```python
from build123d import *

# Parameters (mm, degrees)
BOSS_EXTRU_1_DEPTH      = 75
CONG_1_R                = 5
ESQUISSE2_W             = 12
ESQUISSE2_H             = 27
BOSS_EXTRU_2_DEPTH      = 1.5
ESQUISSE3_R             = 14
ENL_V_MAT_EXTRU_1_DEPTH = 87.989941947
ENL_V_MAT_EXTRU_2_DEPTH = 94.429117653
ENL_V_MAT_EXTRU_3_DEPTH = 89.887569593
ESQUISSE6_R             = 1.2
ENL_V_MAT_EXTRU_4_DEPTH = 20
ESQUISSE7_R             = 1.2
ENL_V_MAT_EXTRU_5_DEPTH = 89.46044325
ESQUISSE9_W             = 15
ESQUISSE9_H             = 10
BOSS_EXTRU_3_DEPTH      = 30
CONG_2_R                = 10
CONG_3_R                = 5
ESQUISSE10_R            = 1.2
ENL_V_MAT_EXTRU_6_DEPTH = 10
ESQUISSE11_R            = 1.2
ENL_V_MAT_EXTRU_7_DEPTH = 15
ESQUISSE12_W            = 12
ESQUISSE12_H            = 2.5
ENL_V_MAT_EXTRU_8_DEPTH = 159.113883129


with BuildPart() as part:
    # Esquisse1 → Boss.-Extru.1 (new, symmetric)
    with BuildSketch(Plane.XY):
        Polygon((-12, 0), (0, 0), (0, 1.5), (5, 1.5), (23, 20), (28, 20), (28, 18.5), (40, 18.5), (40, 12.5), (24.074103459, 12.5), (6.074103459, -6), (-12, -6), align=None)
    extrude(amount=BOSS_EXTRU_1_DEPTH, both=True)

    # Congé1
    cong_1_edges = [part.edges().sort_by_distance(p)[0] for p in [
        (5, 1.5, 0),
        (23, 20, 0),
        (40, 12.5, 0),
        (24.074103459, 12.5, 0),
        (6.074103459, -6, 0),
        (-12, -6, 0),
    ]]
    fillet(cong_1_edges, radius=CONG_1_R)

    # Esquisse2 → Boss.-Extru.2 (add)
    with BuildSketch(Plane(origin=(0, 0, 0), x_dir=(1, 0, 0), z_dir=(0, 1, 0))):
        with Locations((-6, -4)):
            Rectangle(ESQUISSE2_W, ESQUISSE2_H)
    extrude(amount=BOSS_EXTRU_2_DEPTH)

    # Esquisse3 → Enlèv. mat.-Extru.1 (cut, through all)
    with BuildSketch(Plane(origin=(0, 1.5, 0), x_dir=(1, 0, 0), z_dir=(0, 1, 0))):
        with Locations((-14, -4)):
            Circle(ESQUISSE3_R)
    extrude(amount=-ENL_V_MAT_EXTRU_1_DEPTH, mode=Mode.SUBTRACT)

    # Esquisse4 → Enlèv. mat.-Extru.2 (cut, through all)
    with BuildSketch(Plane(origin=(40, 0, 0), x_dir=(0, 0, -1), z_dir=(1, 0, 0))):
        with BuildLine():
            Line((-22, 12), (-18, 9))
            ThreePointArc((-18, 9), (0, 3), (18, 9))
            Line((18, 9), (22, 12))
            ThreePointArc((22, 12), (24.208203932, 14.645898034), (25, 18))
            Line((25, 18), (25, 20))
            Line((25, 20), (-25, 20))
            Line((-25, 20), (-25, 18))
            ThreePointArc((-25, 18), (-24.208203932, 14.645898034), (-22, 12))
        make_face()
    extrude(amount=-ENL_V_MAT_EXTRU_2_DEPTH, mode=Mode.SUBTRACT)

    # Esquisse5 → Enlèv. mat.-Extru.3 (cut, through all)
    with BuildSketch(Plane(origin=(0, 20, 0), x_dir=(1, 0, 0), z_dir=(0, 1, 0))):
        with BuildLine():
            Line((40, 25), (31.163059803, 25))
            ThreePointArc((31.163059803, 25), (26.361328616, 23.849850491), (22.601776236, 20.649033065))
            Line((22.601776236, 20.649033065), (22.601776236, -20.649033065))
            ThreePointArc((22.601776236, -20.649033065), (26.361328616, -23.849850491), (31.163059803, -25))
            Line((31.163059803, -25), (40, -25))
            Line((40, -25), (40, 25))
        make_face()
    extrude(amount=-ENL_V_MAT_EXTRU_3_DEPTH, mode=Mode.SUBTRACT)

    # Esquisse6 → Enlèv. mat.-Extru.4 (cut)
    with BuildSketch(Plane.XY.offset(75)):
        with Locations((25, 16)):
            Circle(ESQUISSE6_R)
        with Locations((5, -2.5)):
            Circle(ESQUISSE6_R)
    enl_v_mat_extru_4 = extrude(amount=-ENL_V_MAT_EXTRU_4_DEPTH, mode=Mode.SUBTRACT)

    # Esquisse7 → Enlèv. mat.-Extru.5 (cut, through all)
    with BuildSketch(Plane(origin=(0, 18.5, 0), x_dir=(1, 0, 0), z_dir=(0, 1, 0))):
        with Locations(Location((35, -55, 0), (0, 0, 180))):
            Circle(ESQUISSE7_R)
        with Locations(Location((-7, -55, 0), (0, 0, 90))):
            Circle(ESQUISSE7_R)
    enl_v_mat_extru_5 = extrude(amount=-ENL_V_MAT_EXTRU_5_DEPTH, mode=Mode.SUBTRACT)

    # Symétrie1: Enlèv. mat.-Extru.4, Enlèv. mat.-Extru.5 across plane
    add(enl_v_mat_extru_4.mirror(Plane.XY), mode=Mode.SUBTRACT)
    add(enl_v_mat_extru_5.mirror(Plane.XY), mode=Mode.SUBTRACT)

    # Esquisse9 → Boss.-Extru.3 (add)
    with BuildSketch(Plane(origin=(0, 0, 0), x_dir=(1, 0, 0), z_dir=(0, 1, 0))):
        with Locations((-14.5, 34.5)):
            Rectangle(ESQUISSE9_W, ESQUISSE9_H)
    extrude(amount=-BOSS_EXTRU_3_DEPTH)

    # Congé2
    cong_2_edges = [part.edges().sort_by_distance(p)[0] for p in [
        (-7, -6, -34.5),
        (-7, -30, -34.5),
    ]]
    fillet(cong_2_edges, radius=CONG_2_R)

    # Congé3
    cong_3_edges = [part.edges().sort_by_distance(p)[0] for p in [
        (-12, -0.5, -39.5),
        (-10.535533906, -4.535533906, -39.5),
        (-2, -6, -39.5),
    ]]
    fillet(cong_3_edges, radius=CONG_3_R)

    # Esquisse10 → Enlèv. mat.-Extru.6 (cut)
    with BuildSketch(Plane.XY.offset(-29.5)):
        with Locations((-18, -24)):
            Circle(ESQUISSE10_R)
        with Locations((-18, -6)):
            Circle(ESQUISSE10_R)
    extrude(amount=-ENL_V_MAT_EXTRU_6_DEPTH, mode=Mode.SUBTRACT)

    # Esquisse11 → Enlèv. mat.-Extru.7 (cut)
    with BuildSketch(Plane(origin=(0, 0, 0), x_dir=(1, 0, 0), z_dir=(0, 1, 0))):
        with Locations(Location((-14, 34.5, 0), (0, 0, 270))):
            Circle(ESQUISSE11_R)
    extrude(amount=-ENL_V_MAT_EXTRU_7_DEPTH, mode=Mode.SUBTRACT)

    # Esquisse12 → Enlèv. mat.-Extru.8 (cut, through all)
    with BuildSketch(Plane.XY.offset(75)):
        with Locations((34, 18.75)):
            Rectangle(ESQUISSE12_W, ESQUISSE12_H)
    extrude(amount=-ENL_V_MAT_EXTRU_8_DEPTH, mode=Mode.SUBTRACT)


solid = part.part
```
Source: CAD feature listing. Evaluate the final solid. Frame: model axes, mm. A direction names the side the tool comes from. Give positions to 0.01 mm unless a question says otherwise; leave off trailing zeros. Write each loop counter-clockwise with the first axis right and the second up, starting at its lowest first coordinate (ties: lowest second). Pieces come first, ordered by that corner, then holes.
1. Section query B-B (y = -12.5). Return the cut outline in (x, z).
2. Section query C-C (z = -14.5). Return the cut outline in (x, y), then the cut area to 3 significant figures.
3. Material intervals for line 1 along Z through (x, y) = (35, 14.5); line 2 along Y through (x, z) = (3, 63); line 3 along X through (y, z) = (14.05, 55), sorted ascending.
4. Access query for faces 1 (the face through (-10, -5, 46)), 2 (the face through (36, 15, 25)), 3 (the face through (-16, -18, -39.5)), 4 (the face through (31, 12.5, 50)). Directions: +Z, -Z, +X, -X, +Y, -Y. A direction counts if a zero-diameter tool reaches every point of the face in a straight line with its end or side. Return the directions, or none.
5. First-contact query: pin 1 (0.5 mm diameter, centred on y = -0.5, z = -19.5, fed in from -X); pin 2 (0.7 mm diameter, centred on x = 5, y = -2.5, fed in from +Z); pin 3 (0.8 mm diameter, centred on y = 0.5, z = 38, fed in from -X). Flat tips, straight axial feed; report the tip coordinate or a pass-through.
6. Pull-direction query (Z, two-part tool) for faces 5 (the face through (-10.01, -27.15, -34.57)), 6 (the face through (23, 14.602, -24.186)), 7 (the face through (-13.5, -0.51, -40.93)); classes: +Z half, -Z half, draft (parallel to the pull), parting line (faces both ways), or undercut.
7. Section query A-A (z = 33). Return the cut outline in (x, y), then the cut area to 3 significant figures.
Output values:
1. outline: (-22, -39.5) - (-6.37, -39.5) - (-6.37, -29.5) - (-22, -29.5) - close; hole circle Ø2.4 at (-14, -34.5)
2. outline: (-12, -1) arc R5 ccw to (-7, -6) - (3.96, -6) arc R5 ccw to (7.55, -4.49) - (18.47, 6.74) - (10.1, 6.74) - (6.47, 3.01) arc R5 cw to (2.89, 1.5) - (0, 1.5) - (0, 0) - (-12, 0) - close
2. area: 183 mm2
3. line 1: z = -75 to -56.2, -53.8 to -25, 25 to 53.8, 56.2 to 75
3. line 2: y = -6 to 1.5
3. line 3: x = 17.21 to 33.8, 36.2 to 38.62
4. face 1: +Z, -X, -Y
4. face 2: +X, +Y, -Y
4. face 3: -Z, -X, -Y
4. face 4: +Z, -Z, +X, -Y
5. pin 1: stops at x = -12
5. pin 2: stops at z = 55
5. pin 3: stops at x = 0
6. face 5: draft
6. face 6: undercut
6. face 7: -Z half
7. outline: (-12, -1) arc R5 ccw to (-7, -6) - (3.96, -6) arc R5 ccw to (7.55, -4.49) - (22.6, 10.99) arc R5 cw to (26.19, 12.5) - (35, 12.5) arc R5 ccw to (40, 17.5) - (28, 17.5) - (28, 20) - (25.11, 20) arc R5 ccw to (21.53, 18.49) - (6.47, 3.01) arc R5 cw to (2.89, 1.5) - (0, 1.5) - (0, 0) - (-12, 0) - close
7. area: 351 mm2
